from build123d import *

# Parameters (mm, degrees)
SKETCH1_W                      = 304.8
SKETCH1_H                      = 355.6
BOSS_EXTRUDE1_DEPTH            = 3.175
F_9_16_0_5625_DIAMETER_HOLE1_D = 14.2875
FILLET1_R                      = 6.35
F_1_4_CLEARANCE_HOLE1_D        = 7.14248
SKETCH2_W                      = 31.75
SKETCH2_H                      = 25.4
CUT_EXTRUDE1_DEPTH             = 4.175
FILLET2_R                      = 1.5875


with BuildPart() as part:
    # Sketch1 → Boss-Extrude1 (new body)
    with BuildSketch(Plane.XY):
        Rectangle(SKETCH1_W, SKETCH1_H)
    extrude(amount=BOSS_EXTRUDE1_DEPTH)

    # 9/16 (0.5625) Diameter Hole1 (through all)
    with Locations(Plane.XY.offset(3.175)):
        with Locations((-127, 162.71875), (-127, 91.28125), (-127, -91.28125), (-127, -162.71875), (127, -162.71875), (127, -91.28125), (127, 91.28125), (127, 162.71875)):
            Hole(F_9_16_0_5625_DIAMETER_HOLE1_D / 2)

    # Fillet1
    fillet1_edges = [part.edges().sort_by_distance(p)[0] for p in [
        (152.4, -177.8, 1.5875),
        (-152.4, -177.8, 1.5875),
        (-152.4, 177.8, 1.5875),
        (152.4, 177.8, 1.5875),
    ]]
    fillet(fillet1_edges, radius=FILLET1_R)

    # 1/4 Clearance Hole1 (through all)
    with Locations(Plane(origin=(0, 0, 0), x_dir=(-1, 0, 0), z_dir=(0, 0, -1))):
        with Locations((-44.45, 56.9515625), (-44.45, -56.9515625), (44.45, 56.9515625), (44.45, -56.9515625)):
            Hole(F_1_4_CLEARANCE_HOLE1_D / 2)

    # Sketch2 → Cut-Extrude1 (cut, through all)
    with BuildSketch(Plane.XY.offset(3.175)):
        with Locations((0, -114.3)):
            Rectangle(SKETCH2_W, SKETCH2_H)
    extrude(amount=-CUT_EXTRUDE1_DEPTH, mode=Mode.SUBTRACT)

    # Fillet2
    fillet2_edges = [part.edges().sort_by_distance(p)[0] for p in [
        (-15.875, -101.6, 1.5875),
        (15.875, -101.6, 1.5875),
        (15.875, -127, 1.5875),
        (-15.875, -127, 1.5875),
    ]]
    fillet(fillet2_edges, radius=FILLET2_R)


solid = part.part
Source: CAD feature listing. Evaluate the final solid. Frame: model axes, mm. Give positions to 0.01 mm unless a question says otherwise; leave off trailing zeros. Write each loop counter-clockwise with the first axis right and the second up, starting at its lowest first coordinate (ties: lowest second). Pieces come first, ordered by that corner, then holes. Notation, with made-up numbers: M 12.25,24 L 20.25,24 A30 ccw 20.25,58 Z; hole C 68,49.5 d1. An arc over 180 degrees is marked long. Return JSON: item names as keys, results as strings. Group by question number.
1) Material intervals for line 1 along Y through (x, z) = (127, 2.05) (1 decimal); line 2 along X through (y, z) = (-110, 1.85) (3 decimals); line 3 along X through (y, z) = (-55, 3.05), sorted ascending. Write a range as [from, to].
2) Pull-direction query (X, two-part tool) for faces 1 (the face through (-2, 2, 0)), 2 (the face through (134.137, -90.967, 1.565)); classes: pulls with the +X half, pulls with the -X half, needs draft (parallel to the pull), parting line crosses it, or undercut.
3) Cut plane A-A, the plane y = -110.5. Output: boundary loops of the cut face in (x, z) (3 decimals).
4) Cut plane C-C, the plane z = 1.35. Give the number of separate pieces and of enclosed holes in the cut face, plus the area to 3 significant figures.
5) Cut plane B-B, the plane x = 127. Output: boundary loops of the cut face in (y, z) (1 decimal), plus the area to 3 significant figures.
6) Pin query (flat end, axial travel): P1, Ø11.5, axis at x = 127, y = 162.72, coming from the +Z side. Return the tip coordinate at first contact, or that it passes through.
Recorded:
{
 "1": {"line 1": "y = [-177.8, -169.9], [-155.6, -98.4], [-84.1, 84.1], [98.4, 155.6], [169.9, 177.8]", "line 2": "x = [-152.4, -15.875], [15.875, 152.4]", "line 3": "x = [-152.4, -47.44], [-41.46, 41.46], [47.44, 152.4]"},
 "2": {"face 1": "needs draft", "face 2": "undercut"},
 "3": {"outline": "M -152.4,0 L -15.875,0 L -15.875,3.175 L -152.4,3.175 Z; M 15.875,0 L 152.4,0 L 152.4,3.175 L 15.875,3.175 Z"},
 "4": {"separate pieces": "1", "enclosed holes": "13", "area": "106,000 mm²"},
 "5": {"outline": "M -177.8,0 L -169.9,0 L -169.9,3.2 L -177.8,3.2 Z; M -155.6,0 L -98.4,0 L -98.4,3.2 L -155.6,3.2 Z; M -84.1,0 L 84.1,0 L 84.1,3.2 L -84.1,3.2 Z; M 98.4,0 L 155.6,0 L 155.6,3.2 L 98.4,3.2 Z; M 169.9,0 L 177.8,0 L 177.8,3.2 L 169.9,3.2 Z", "area": "948 mm²"},
 "6": {"P1": "passes through"}
}
